```python
from build123d import *

# Parameters (mm, degrees)
ESQUISSE1_R             = 6
BOSS_EXTRU_1_DEPTH      = 6
BOSS_EXTRU_1_TAPER      = 15
ESQUISSE2_R             = 3
ENL_V_MAT_EXTRU_1_DEPTH = 2.5
D_GAGEMENT_M31_D        = 3.4


with BuildPart() as part:
    # Esquisse1 → Boss.-Extru.1 (new body)
    with BuildSketch(Plane(origin=(0, 0, 0), x_dir=(1, 0, 0), z_dir=(0, 1, 0))):
        Circle(ESQUISSE1_R)
    extrude(amount=BOSS_EXTRU_1_DEPTH, taper=BOSS_EXTRU_1_TAPER)

    # Esquisse2 → Enlèv. mat.-Extru.1 (cut)
    with BuildSketch(Plane(origin=(0, 6, 0), x_dir=(1, 0, 0), z_dir=(0, 1, 0))):
        with Locations(Location((0, 0, 0), (0, 0, 270))):
            Circle(ESQUISSE2_R)
    extrude(amount=-ENL_V_MAT_EXTRU_1_DEPTH, mode=Mode.SUBTRACT)

    # Dégagement M31 (through all)
    with Locations(Plane(origin=(0, 3.5, 0), x_dir=(1, 0, 0), z_dir=(0, 1, 0))):
        with Locations((0, 0)):
            Hole(D_GAGEMENT_M31_D / 2)


solid = part.part
```
Source: CAD feature listing. Evaluate the final solid. Frame: model axes, mm. A direction names the side the tool comes from. Coordinates: 2 decimals unless noted, no trailing zeros. Loops run counter-clockwise (first coordinate to the right, second up) from the corner with the lowest first, then second, coordinate; pieces in that order, holes last. Notation, with made-up numbers: M 48,-15 L 89,-15 A22 cw 89,17 Z; hole C 24,-40 d1. An arc over 180 degrees is marked long. Put each result on its own line as item: value. Start each with the question number.
1) Pull-direction query (X, two-part tool) for faces 1 (the face through (3, 6, 1)), 2 (the face through (-2, 3.5, 0)), 3 (the face through (4.605, 4.375, -1.45)); classes: pulls with the +X half, pulls with the -X half, needs draft (parallel to the pull), parting line crosses it, or undercut.
2) Reachability of faces 4 (the face through (0.9, 4.77, 2.86)), 5 (the face through (1.25, 0, -1.42)) from +Z, -Z, +X, -X, +Y, -Y: full face, straight path, thin tool, end or side. Return the list, or none.
3) Cut plane C-C on y = 1.75. Return the cut outline in (x, z).
4) Cut plane A-A on x = 0. Return the cut outline in (y, z), then the cut area to 3 significant figures.
5) Contact query for flat-ended pins moving along their axis: pin 1 Ø6.5 at (x, z) = (-1, 0) entering from +Y; pin 2 Ø3 at (y, z) = (4.5, 3.5) entering from +X; pin 3 Ø3 at (y, z) = (2, 0) entering from -X; pin 4 Ø1.5 at (x, y) = (-0.5, 1.5) entering from +Z. Output: stop coordinate, or through.
6) Ray query, L1, parallel to Y at x = -1, z = -2.75; L2, parallel to X at y = 2, z = -3.25; L3, parallel to Z at x = 0, y = 1.25. Return the intervals inside material, ascending. Write a range as from..to.
7) Cut plane B-B on y = 2.5. Return the cut outline in (x, z), then the cut area to 3 significant figures.
The answers:
1. face 1: needs draft
1. face 2: undercut
1. face 3: parting line crosses it
2. face 4: +Y
2. face 5: +Z, -Z, +X, -X, -Y
3. outline: C 0,0 d11.06; hole C 0,0 d3.4
4. outline: M 0,-6 L 6,-4.39 L 6,-3 L 3.5,-3 L 3.5,-1.7 L 0,-1.7 Z; M 0,1.7 L 3.5,1.7 L 3.5,3 L 6,3 L 6,4.39 L 0,6 Z
4. area: 35.5 mm²
5. pin 1: stops at y = 6
5. pin 2: stops at x = 4.48
5. pin 3: stops at x = -5.87
5. pin 4: stops at z = 5.78
6. L1: y = 0..3.5
6. L2: x = -4.39..4.39
6. L3: z = -5.67..-1.7, 1.7..5.67
7. outline: C 0,0 d10.66; hole C 0,0 d3.4
7. area: 80.2 mm²
